Read the model definition and answer for the solid it produces. Units are mm, in the model's axes. A direction names the side the tool comes from. Coordinates: 2 decimals unless noted, no trailing zeros. Write each loop counter-clockwise with the first axis right and the second up, starting at its lowest first coordinate (ties: lowest second). Pieces come first, ordered by that corner, then holes. Notation, with made-up numbers: (69, -25) -> (127, -25) arc R13 ccw to (127, -21) -> close; hole circle Ø3 at (-36, -27.5). An arc over 180 degrees is marked (long way). Answer in a Markdown table with one row per item. Add a question column.
Item 1: Section A-A on y = 15 is taken. Write down the section's boundary in (x, z), then the cut area to 3 significant figures.
Item 2: Section C-C on z = 1.15 is taken. Write down the section's boundary in (x, y).
Item 3: Section D-D on x = -3.25 is taken. Write down the section's boundary in (y, z), then the cut area to 3 significant figures.
Item 4: Given pin 1 Ø3 at (x, z) = (0.5, 1) entering from -Y; pin 2 Ø2 at (x, z) = (-4.5, 3) entering from +Y; pin 3 Ø5 at (x, y) = (-1, 29.5) entering from +Z, each flat-ended and moving along its own axis, determine where each tip first touches the part or whether it passes through.
Item 5: Which of the six approach directions +Z, -Z, +X, -X, +Y, -Y give full straight-line access (tool end or side, diameter ignored) to faces 1 (the face through (0, 34, 4)), 2 (the face through (-8.08, 21, 1))?
Item 6: Straight lines are drawn through the part: line 1 (Y direction, x = 1, z = 0.7); line 2 (Y direction, x = 0, z = 1); line 3 (Z direction, x = -5.5, y = 19.5). For each, find the intervals that lie inside material, in ascending order. Write a range as from..to.
Item 7: Section B-B on x = 0 is taken. Write down the section's boundary in (y, z), then the cut area to 3 significant figures.
Item 8: For a pull along X with two mould halves and no side action, classify faces 3 (the face through (8.08, -5, 1)), 4 (the face through (1.61, 25.44, 0.99)), 5 (the face through (-5, -8.08, 1)) as +X half, -X half, draft (parallel to the pull), parting line (faces both ways), or undercut.
Autodesk Inventor part; units mm, degrees
ref_plane "Work Plane1" through (8.08, 0, 0) normal (1, 0, 0) x (0, 1, 0)
ref_plane "Work Plane2" through (-8.08, 0, 0) normal (1, 0, 0) x (0, 1, 0)
ref_plane "Work Plane3" through (0, -8.08, 0) normal (0, 1, 0) x (-1, 0, 0)
sketch "Sketch1" plane through (0, 0, 0) normal (0, 0, 1) x (1, 0, 0)
  circle A0 centre (0, 0) radius 36
  dimension "d0" = 72
extrude "Extrusion1" add sketch "Sketch1" along normal blind 2
sketch "Sketch2" plane through (0, 0, 2) normal (0, 0, 1) x (1, 0, 0)
  circle A0 centre (0, 0) radius 36
  circle A1 centre (0, 0) radius 34
  dimension "d3" = 2
extrude "Extrusion2" add sketch "Sketch2" along normal blind 4
sketch "Sketch4" plane through (0, 0, 2) normal (0, 0, 1) x (1, 0, 0)
  point P0 (0, 0)
  point P1 (0, 0)
hole "Hole1" at (0, 0, 2) direction (0, 0, -1) diameter 10.1 end through all
sketch "Sketch5" plane through (0, 0, 2) normal (0, 0, 1) x (1, 0, 0)
  point P0 (0, 0)
  point P1 (0, 23.3333)
  dimension "d13" = 23.3333
hole "Hole2" at (0, 23.3333, 2) direction (0, 0, -1) diameter 5.3 end through all
pattern_circular "Circular Pattern1" count 5 over 360 about axis through (0, 0, -100) along (0, 0, 1) of "Hole2"
sketch "Sketch8" plane through (0, 0, 2) normal (0, 0, 1) x (1, 0, 0)
  circle A0 centre (22.1913, 7.2104) radius 2.65
  circle A1 centre (13.715, -18.8771) radius 2.65
  circle A2 centre (-13.715, -18.8771) radius 2.65
  circle A3 centre (-22.1913, 7.2104) radius 2.65
  circle A4 centre (0, 23.3333) radius 2.65
  circle A5 centre (0, 0) radius 5.05
  circle A6 centre (0, 0) radius 34
  line L0 (-2, 16) -> (2, 16)
  line L1 (2, 16) -> (2, 8)
  line L2 (2, 8) -> (-2, 8)
  line L3 (-2, 8) -> (-2, 16)
  dimension "d43" = 4
  dimension "d44" = 8
  dimension "d45" = 8
  dimension "d48" = 2
extrude "Extrusion5" cut sketch "Sketch8" against normal up to surface (2 mm away) draft 2 contours L0 L1 L2 L3
fillet "Fillet2" radius 0.25 4 edges at (0, 7.9302, 0) (2.0698, 12, 0) (0, 16.0698, 0) (-2.0698, 12, 0)
pattern_circular "Circular Pattern3" count 4 over 360 about axis through (0, 0, -100) along (0, 0, 1) of "Extrusion5", "Fillet2"
ref_plane "Work Plane1" through (8.08, 0, 0) normal (1, 0, 0) x (0, 1, 0)
ref_plane "Work Plane2" through (-8.08, 0, 0) normal (1, 0, 0) x (0, 1, 0)
ref_plane "Work Plane3" through (0, -8.08, 0) normal (0, 1, 0) x (-1, 0, 0)
split "Split1" plane through (0, -8.08, 0) removes the side toward (0, -1, 0)
split "Split2" plane through (8.08, 0, 0) removes the side toward (1, 0, 0)
split "Split3" plane through (-8.08, 0, 0) removes the side toward (-1, 0, 0)
equation "\"d0\" = W_innerDiameter + W_wallThickness"
equation "\"d1\" = W_wallThickness"
equation "\"d3\" = W_wallThickness"
equation "\"d4\" = W_innerDepth"
equation "\"d6\" = W_innerGearHoleDiameter"
equation "\"d14\" = W_outerGearHoleDiameter"
equation "\"W_wallThickness\" = 2"
equation "\"W_innerDepth\" = 4"
equation "\"W_innerGearHoleDiameter\" = 10.1"
equation "\"W_outerGearHoleDiameter\" = 5.3"
equation "\"OG_distanceFromCenter\" = 23.33333"
equation "\"W_innerDiameter\" = 70"
equation "\"Wheel_Related_W_\" = 0"
equation "\"W_holesClearance\" = 0.3"
equation "\"TempSpotReserved7\" = 0"
equation "\"TempSpotReserved8\" = 0"
equation "\"TempSpotReserved9\" = 0"
equation "\"TempSpotReserved10\" = 0"
equation "\"TempSpotReserved11\" = 0"
equation "\"TempSpotReserved12\" = 0"
equation "\"TempSpotReserved13\" = 0"
equation "\"TempSpotReserved14\" = 0"
equation "\"TempSpotReserved15\" = 0"
equation "\"TempSpotReserved16\" = 0"
equation "\"TempSpotReserved17\" = 0"
equation "\"TempSpotReserved18\" = 0"
equation "\"TempSpotReserved19\" = 0"
equation "\"TempSpotReserved20\" = 0"
equation "\"Inner_Gear_Related_IG_\" = 0"
equation "\"IG_shaftDiameter\" = 7.5"
equation "\"IG_shaftLength\" = 15"
equation "\"IG_gearThickness\" = 2"
equation "\"TempSpotReserved25\" = 0"
equation "\"TempSpotReserved26\" = 0"
equation "\"TempSpotReserved27\" = 0"
equation "\"TempSpotReserved28\" = 0"
equation "\"TempSpotReserved29\" = 0"
equation "\"TempSpotReserved30\" = 0"
equation "\"TempSpotReserved31\" = 0"
equation "\"TempSpotReserved32\" = 0"
equation "\"TempSpotReserved33\" = 0"
equation "\"TempSpotReserved34\" = 0"
equation "\"TempSpotReserved35\" = 0"
equation "\"TempSpotReserved36\" = 0"
equation "\"TempSpotReserved37\" = 0"
equation "\"TempSpotReserved38\" = 0"
equation "\"TempSpotReserved39\" = 0"
equation "\"TempSpotReserved40\" = 0"
equation "\"Outer_Gear_Related_OG_\" = 0"
equation "\"OG_shaftDiameter\" = 5"
equation "\"OG_gearDiameter\" = 26.66667"
equation "\"OG_shaftLength\" = 7"
equation "\"OG_gearThickness\" = 2"
equation "\"TempSpotReserved47\" = 0"
equation "\"TempSpotReserved48\" = 0"
equation "\"TempSpotReserved49\" = 0"
equation "\"TempSpotReserved50\" = 0"
equation "\"TempSpotReserved51\" = 0"
equation "\"TempSpotReserved52\" = 0"
equation "\"TempSpotReserved53\" = 0"
equation "\"TempSpotReserved54\" = 0"
equation "\"TempSpotReserved55\" = 0"
equation "\"TempSpotReserved56\" = 0"
equation "\"TempSpotReserved57\" = 0"
equation "\"TempSpotReserved58\" = 0"
equation "\"TempSpotReserved59\" = 0"
equation "\"TempSpotReserved60\" = 0"
equation "\"Leg_Extensions_Related_LE_\" = 0"
equation "\"LE_baseDiameter\" = 5"
equation "\"LE_maxLength\" = 24.6522"
equation "\"LE_thickness\" = 2.5"
equation "\"IG_ratioToOuterGear\" = 0.75"
equation "\"B_bearingThickness\" = 1"
equation "\"TempSpotReserved43\" = 0"
equation "\"TempSpotReserved45\" = 0"
equation "\"Thisisatest\" = 25.4"
equation "\"TempSpotReserved46\" = 0"
equation "\"TempSpotReserved44\" = 0"
equation "\"LE_offsetAboveOuterGear\" = 0"
equation "\"Bearing_Related_B_\" = 0"
equation "\"TempSpotReserved42\" = 0"
equation "\"OG_skirtOffset\" = 1"
equation "\"OG_skirtThickness\" = 1"
equation "\"IG_skirtThickness\" = 2"
equation "\"IG_extentionLength\" = 18.33333"
equation "\"IG_extentionThickness\" = 3"
equation "\"IG_slitWidth\" = 4"
equation "\"IG_slitlength\" = 8"
equation "\"IG_slitClearance\" = 0.2"
equation "\"IG_slitDistanceFromCenterHole\" = 8"
equation "\"Reserved_10\" = 0"
equation "\"Reserved_9\" = 0"
equation "\"Reserved_11\" = 0"
equation "\"Reserved_12\" = 0"
equation "\"Reserved_8\" = 0"
equation "\"Reserved_7\" = 0"
equation "\"Reserved_26\" = 0"
equation "\"Reserved_20\" = 0"
equation "\"Reserved_22\" = 0"
equation "\"Reserved_23\" = 0"
equation "\"Reserved_25\" = 0"
equation "\"Reserved_24\" = 0"
equation "\"Reserved_21\" = 0"
equation "\"Reserved_19\" = 0"
equation "\"Reserved_27\" = 0"
equation "\"Reserved_14\" = 0"
equation "\"Reserved_15\" = 0"
equation "\"Reserved_16\" = 0"
equation "\"Reserved_13\" = 0"
equation "\"Reserved_17\" = 0"
equation "\"Reserved_18\" = 0"
equation "\"Bearing_Related_BR_\" = 0"
equation "\"BR_bearingThickness\" = 1"
equation "\"Block_Related_BL_\" = 0"
equation "\"BL_width\" = 3.8"
equation "\"BL_length\" = 7.8"
equation "\"W_filletRadius\" = 0.25"
equation "\"W_extrutsionTaperAngle\" = 2deg"
equation "\"OG_protrudeDistance\" = 3"
properties part number "wheel1"
Results below:
| question | item | result |
|---|---|---|
| 1 | outline | (-8.08, 0) -> (-2.31, 0) arc R0.25 ccw to (-2.06, 0.24) -> (-2, 2) -> (-8.08, 2) -> close; (2, 2) -> (2.06, 0.24) arc R0.25 ccw to (2.31, 0) -> (8.08, 0) -> (8.08, 2) -> close |
| 1 | area | 24.2 mm2 |
| 2 | outline | (-8.08, -8.08) -> (-2.03, -8.08) -> (-2.03, -7.97) -> (2.03, -7.97) -> (2.03, -8.08) -> (8.08, -8.08) -> (8.08, -2.03) -> (7.97, -2.03) -> (7.97, 2.03) -> (8.08, 2.03) -> (8.08, 35.08) arc R36 ccw to (-8.08, 35.08) -> (-8.08, 2.03) -> (-7.97, 2.03) -> (-7.97, -2.03) -> (-8.08, -2.03) -> close; hole circle Ø10.1 at (0, 0); hole circle Ø5.3 at (0, 23.33); hole (-2.03, 7.97) -> (2.03, 7.97) -> (2.03, 16.03) -> (-2.03, 16.03) -> close |
| 3 | outline | (-8.08, 0) -> (-3.87, 0) -> (-3.87, 2) -> (-8.08, 2) -> close; (3.87, 0) -> (35.85, 0) -> (35.85, 6) -> (33.84, 6) -> (33.84, 2) -> (3.87, 2) -> close |
| 3 | area | 80.4 mm2 |
| 4 | pin 1 | stops at y = -8 |
| 4 | pin 2 | stops at y = 35.83 |
| 4 | pin 3 | stops at z = 2 |
| 5 | face 1 | +Z, -Y |
| 5 | face 2 | +Z, -Z, -X, +Y, -Y |
| 6 | line 1 | y = -7.95..-4.95, 4.95..7.95, 16.05..20.88, 25.79..35.99 |
| 6 | line 2 | y = -7.97..-5.05, 5.05..7.97, 16.03..20.68, 25.98..36 |
| 6 | line 3 | z = 0..2 |
| 7 | outline | (-8, 2) -> (-7.94, 0.24) arc R0.25 ccw to (-7.69, 0) -> (-5.05, 0) -> (-5.05, 2) -> close; (5.05, 0) -> (7.69, 0) arc R0.25 ccw to (7.94, 0.24) -> (8, 2) -> (5.05, 2) -> close; (16, 2) -> (16.06, 0.24) arc R0.25 ccw to (16.31, 0) -> (20.68, 0) -> (20.68, 2) -> close; (25.98, 0) -> (36, 0) -> (36, 6) -> (34, 6) -> (34, 2) -> (25.98, 2) -> close |
| 7 | area | 49.0 mm2 |
| 8 | face 3 | +X half |
| 8 | face 4 | undercut |
| 8 | face 5 | draft |
